from build123d import *

# Parameters (mm, degrees)
SKETCH2_R          = 3
CUT_EXTRUDE1_DEPTH = 9
CIRPATTERN1_COUNT  = 4


with BuildPart() as part:
    # Sketch1 → Revolve1 (revolve)
    with BuildSketch(Plane.XY, mode=Mode.PRIVATE) as revolve1_sk:
        Polygon((-2, 7.705702305), (-2, -7.705702305), (-14.25, -10.988079912), (-14.25, 9.011920088), (-2.35, 9.011920088), align=None)
    revolve(revolve1_sk.sketch.rotate(Axis((0, 20.798274686, 0), (0, -1, 0)), 270), axis=Axis((0, 20.798274686, 0), (0, -1, 0)))

    # Sketch2 → Cut-Extrude1 (cut)
    with BuildSketch(Plane(origin=(14.25, 0, 0), x_dir=(0, 0, -1), z_dir=(1, 0, 0))):
        with Locations((0, -0.988079912)):
            Circle(SKETCH2_R)
    cut_extrude1 = extrude(amount=-CUT_EXTRUDE1_DEPTH, mode=Mode.SUBTRACT)

    # CirPattern1: Cut-Extrude1 ×4 about axis
    cirpattern1_axis = Axis((0, 0, 0), (0, 1, 0))
    for i in range(1, CIRPATTERN1_COUNT):
        add(cut_extrude1.rotate(cirpattern1_axis, i * 360 / CIRPATTERN1_COUNT), mode=Mode.SUBTRACT)


solid = part.part
Verification items for the finished model (mm, model axes). A direction names the side the tool comes from. Give positions to 0.01 mm unless a question says otherwise; leave off trailing zeros. Loops run counter-clockwise (first coordinate to the right, second up) from the corner with the lowest first, then second, coordinate; pieces in that order, holes last.
1) Set-up check for faces 1 (the cylindrical face through (2.381, -2.814, -9.813)), 2 (the flat face through (0, -1, 5.25)), 3 (the flat face through (-5.25, -1, 0)), 4 (the cylindrical face through (9.813, -3.917, 0.65)): record each of +Z, -Z, +X, -X, +Y, -Y from which the full face is reachable in a straight line by a thin tool's end or side.
2) Sectioned sample at D-D, the plane y = 1. Enter the section's corners in (x, z).
3) Draft check along Z on faces 5 (the cylindrical face through (5.458, -0.848, 13.163)), 6 (the cylindrical face through (-0.65, -3.917, 9.813)), 7 (the flat face through (0, -1, -5.25)), 8 (the cylindrical face through (-9.813, -3.917, -0.65)). Enter one of: pulls with the +Z half, pulls with the -Z half, needs draft (parallel to the pull), parting line crosses it, or undercut.
4) Depth check by flat-ended pin: pin 1 Ø6 at (y, z) = (-2, -4.5) entering from -X; pin 2 Ø1.5 at (x, y) = (-3, 3) entering from -Z; pin 3 Ø1.8 at (x, y) = (0, -0.5) entering from +Z. Enter the tip coordinate at first touch or a pass-through.
5) Sectioned sample at A-A, the plane z = 0. Enter the section's corners in (x, y).
6) Sectioned sample at B-B, the plane x = 0. Enter the section's corners in (y, z), then the cut area to 3 significant figures.
7) Thickness scan on line 1 along X through (y, z) = (-2.75, 0); line 2 along X through (y, z) = (7.25, -0.5); line 3 along Y through (x, z) = (9.5, 1). Record the ranges inside material, lowest first.
8) Sectioned sample at C-C, the plane y = 6.25. Enter the section's corners in (x, z).
Answers:
1. face 1: -Z
1. face 2: +Z
1. face 3: -X
1. face 4: +X
2. outline: (-14.07, -2.25) arc R14.25 ccw to (-2.25, -14.07) - (-2.25, -5.25) - (2.25, -5.25) - (2.25, -14.07) arc R14.25 ccw to (14.07, -2.25) - (5.25, -2.25) - (5.25, 2.25) - (14.07, 2.25) arc R14.25 ccw to (2.25, 14.07) - (2.25, 5.25) - (-2.25, 5.25) - (-2.25, 14.07) arc R14.25 ccw to (-14.07, 2.25) - (-5.25, 2.25) - (-5.25, -2.25) - close; hole circle Ø4 at (0, 0)
3. face 5: parting line crosses it
3. face 6: needs draft
3. face 7: pulls with the -Z half
3. face 8: undercut
4. pin 1: stops at x = -14.13
4. pin 2: stops at z = -14.07
4. pin 3: stops at z = 5.25
5. outline: (-14.25, -10.99) - (-2, -7.71) - (-2, 7.71) - (-2.35, 9.01) - (-14.25, 9.01) - (-14.25, 2.01) - (-5.25, 2.01) - (-5.25, -3.99) - (-14.25, -3.99) - close; (2, -7.71) - (14.25, -10.99) - (14.25, -3.99) - (5.25, -3.99) - (5.25, 2.01) - (14.25, 2.01) - (14.25, 9.01) - (2.35, 9.01) - (2, 7.71) - close
6. outline: (-10.99, -14.25) - (-3.99, -14.25) - (-3.99, -5.25) - (2.01, -5.25) - (2.01, -14.25) - (9.01, -14.25) - (9.01, -2.35) - (7.71, -2) - (-7.71, -2) - close; (-10.99, 14.25) - (-7.71, 2) - (7.71, 2) - (9.01, 2.35) - (9.01, 14.25) - (2.01, 14.25) - (2.01, 5.25) - (-3.99, 5.25) - (-3.99, 14.25) - close
6. area: 341 mm2
7. line 1: x = -5.25 to -2, 2 to 5.25
7. line 2: x = -14.24 to -1.94, 1.94 to 14.24
7. line 3: y = -9.73 to -3.82, 1.84 to 9.01
8. outline: circle Ø28.5 at (0, 0); hole circle Ø4 at (0, 0)
